Could you check a few things on this drawing? It's one solid part, dimensions in mm from its lowest x, y, z. A direction names the side the tool comes from. Round coordinates to 2 decimals unless told otherwise and drop trailing zeros. Write each loop counter-clockwise with the first axis right and the second up, starting at its lowest first coordinate (ties: lowest second). Pieces come first, ordered by that corner, then holes. Notation, with made-up numbers: (72.5, -4.75) - (128.5, -4.75) arc R31 ccw to (128.5, 21.25) - close; hole circle Ø6 at (65, 64.25). An arc over 180 degrees is marked (long way). One line per question, with ' | ' between items. Start each with the question number.
(1) Imagine slicing it at A-A (x = 8.5). Write out the boundary of the cut face in (y, z), plus the area to 3 significant figures.
(2) Will these pins go through, and if not, where does the flat tip stop? pin 1 (10 mm diameter, centred on x = 70, y = 5.5, fed in from -Z); pin 2 (4 mm diameter, centred on x = 23.5, z = 12, fed in from +Y); pin 3 (2.5 mm diameter, centred on x = 67, y = 2.5, fed in from +Z); pin 4 (1.5 mm diameter, centred on x = 69.5, z = 6, fed in from -Y).
(3) Thinking about a two-plate mould opening in X: for the marked faces 1, 2 and 3, which applies, pulls with the +X half, pulls with the -X half, needs draft (parallel to the pull), parting line crosses it, or undercut?
(4) Imagine slicing it at B-B (y = 15). Write out the boundary of the cut face in (x, z).
(5) Imagine slicing it at C-C (z = 9). Write out the boundary of the cut face in (x, y).
(6) If I drill on L1, parallel to Y at x = 75.5, z = 4; L2, parallel to X at y = 22.5, z = 14.5; L3, parallel to Y at x = 75.5, z = 6.5, over which ranges is the centre line in solid material (lowest first)?
(7) Imagine slicing it at D-D (x = 75.5). Write out the boundary of the cut face in (y, z), plus the area to 4 significant figures.
(8) For the marked faces 4, 5 and 6, which set-ups out of +Z, -Z, +X, -X, +Y, -Y let a thin tool reach every point of the face, with its end or its side?
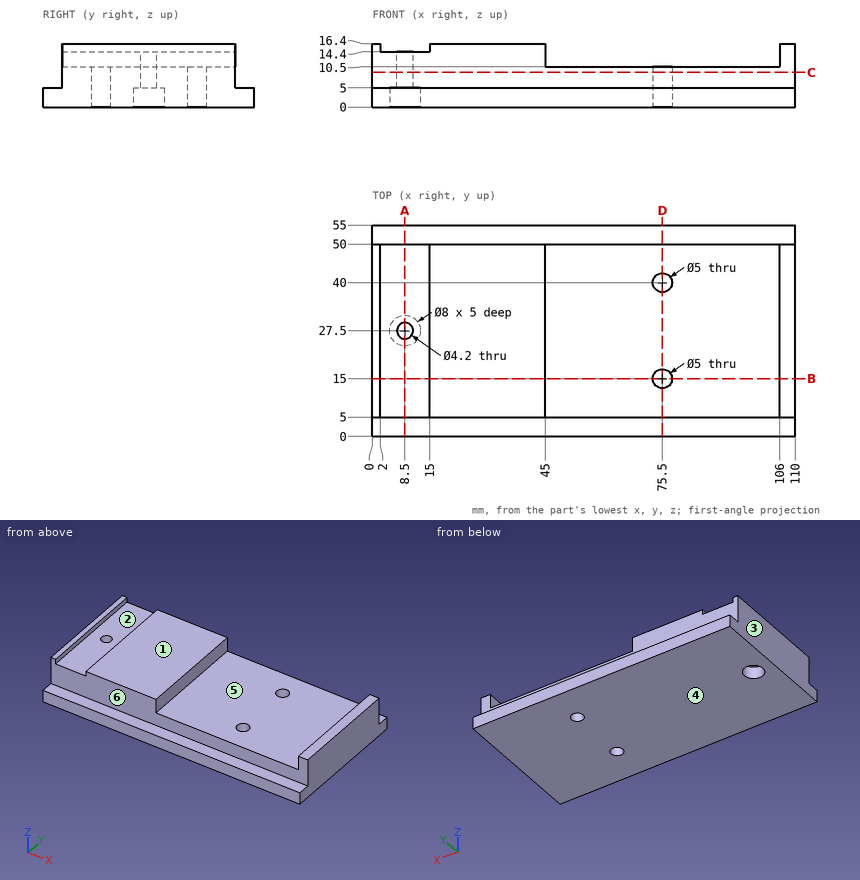
Check sheet entries:
1) outline: (0, 0) - (23.5, 0) - (23.5, 5) - (25.4, 5) - (25.4, 14.4) - (5, 14.4) - (5, 5) - (0, 5) - close; (29.6, 5) - (31.5, 5) - (31.5, 0) - (55, 0) - (55, 5) - (50, 5) - (50, 14.4) - (29.6, 14.4) - close | area: 619 mm^2
2) pin 1: z = 0 | pin 2: y = 50 | pin 3: z = 5 | pin 4: y = 5
3) face 1: needs draft | face 2: undercut | face 3: pulls with the -X half
4) outline: (0, 0) - (73, 0) - (73, 10.5) - (45, 10.5) - (45, 16.4) - (15, 16.4) - (15, 14.4) - (2, 14.4) - (2, 16.4) - (0, 16.4) - close; (78, 0) - (110, 0) - (110, 16.4) - (106, 16.4) - (106, 10.5) - (78, 10.5) - close
5) outline: (0, 5) - (110, 5) - (110, 50) - (0, 50) - close; hole circle Ø4.2 at (8.5, 27.5); hole circle Ø5 at (75.5, 15); hole circle Ø5 at (75.5, 40)
6) L1: 0 to 12.5, 17.5 to 37.5, 42.5 to 55 | L2: 0 to 2, 15 to 45, 106 to 110 | L3: 5 to 12.5, 17.5 to 37.5, 42.5 to 50
7) outline: (0, 0) - (12.5, 0) - (12.5, 10.5) - (5, 10.5) - (5, 5) - (0, 5) - close; (17.5, 0) - (37.5, 0) - (37.5, 10.5) - (17.5, 10.5) - close; (42.5, 0) - (55, 0) - (55, 5) - (50, 5) - (50, 10.5) - (42.5, 10.5) - close | area: 417.5 mm^2
8) face 4: -Z, +X, -X, +Y, -Y | face 5: +Z, +Y, -Y | face 6: +Z, +X, -X, -Y
